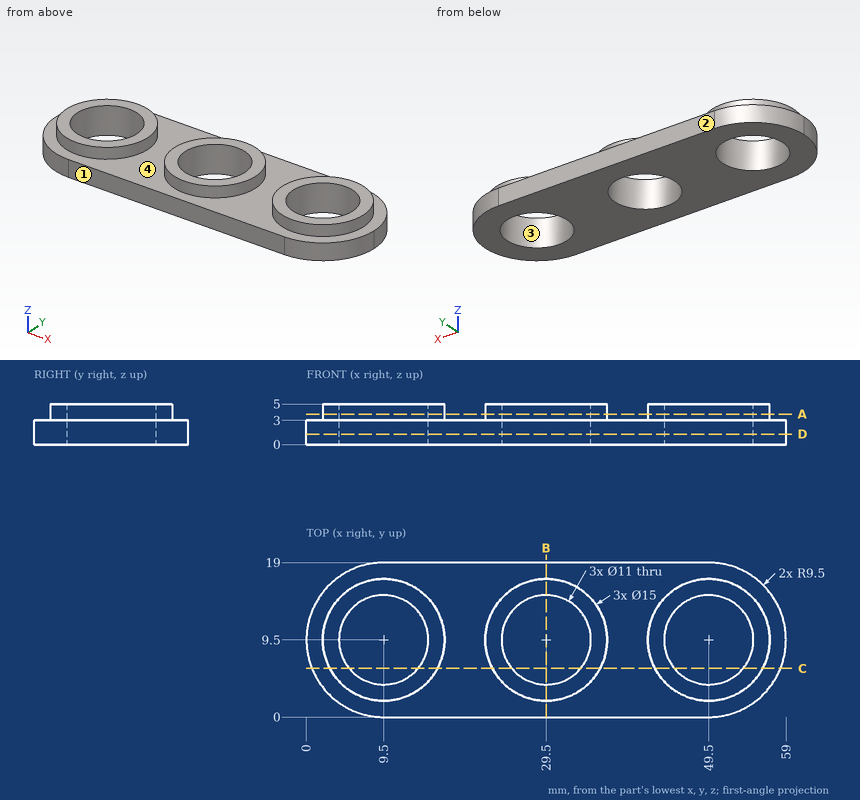
Geometry check sheet. Reference: drawing and pictorial views, mm from the part's lowest x, y, z. Round coordinates to 2 decimals unless told otherwise and drop trailing zeros. Write each loop counter-clockwise with the first axis right and the second up, starting at its lowest first coordinate (ties: lowest second). Pieces come first, ordered by that corner, then holes.
Item 1: Section check D-D (z = 1.3). Record the boundary of the cut face in (x, y), plus the area to 3 significant figures.
Determined:
outline: (9.5, 0) - (49.5, 0) arc R9.5 ccw to (49.5, 19) - (9.5, 19) arc R9.5 ccw to start; hole circle Ø11 at (9.5, 9.5); hole circle Ø11 at (29.5, 9.5); hole circle Ø11 at (49.5, 9.5)
area: 758 mm2
Item 2: Mould release check, pull along Y, two halves, no side actions. Record for the marked faces 1, 2, 3 and 4: +Y half, -Y half, draft (parallel to the pull), parting line (faces both ways), or undercut.
Determined:
face 1: -Y half
face 2: +Y half
face 3: undercut
face 4: draft
Item 3: Section check B-B (x = 29.5). Record the boundary of the cut face in (y, z).
Determined:
outline: (0, 0) - (4, 0) - (4, 5) - (2, 5) - (2, 3) - (0, 3) - close; (15, 0) - (19, 0) - (19, 3) - (17, 3) - (17, 5) - (15, 5) - close
Item 4: Section check C-C (y = 6). Record the boundary of the cut face in (x, z), plus the area to 3 significant figures.
Determined:
outline: (0.67, 0) - (5.26, 0) - (5.26, 5) - (2.87, 5) - (2.87, 3) - (0.67, 3) - close; (13.74, 0) - (25.26, 0) - (25.26, 5) - (22.87, 5) - (22.87, 3) - (16.13, 3) - (16.13, 5) - (13.74, 5) - close; (33.74, 0) - (45.26, 0) - (45.26, 5) - (42.87, 5) - (42.87, 3) - (36.13, 3) - (36.13, 5) - (33.74, 5) - close; (53.74, 0) - (58.33, 0) - (58.33, 3) - (56.13, 3) - (56.13, 5) - (53.74, 5) - close
area: 125 mm2
Item 5: Material ranges on line 1 along Y through (x, z) = (9.5, 2.8); line 2 along X through (y, z) = (5.5, 4.05); line 3 along X through (y, z) = (6.25, 3.65), recorded low to high.
Determined:
line 1: y = 0 to 4, 15 to 19
line 2: x = 3.16 to 5.73, 13.27 to 15.84, 23.16 to 25.73, 33.27 to 35.84, 43.16 to 45.73, 53.27 to 55.84
line 3: x = 2.74 to 5.06, 13.94 to 16.26, 22.74 to 25.06, 33.94 to 36.26, 42.74 to 45.06, 53.94 to 56.26
Item 6: Section check A-A (z = 3.75). Record the boundary of the cut face in (x, y).
Determined:
outline: circle Ø15 at (9.5, 9.5); circle Ø15 at (29.5, 9.5); circle Ø15 at (49.5, 9.5); hole circle Ø11 at (9.5, 9.5); hole circle Ø11 at (29.5, 9.5); hole circle Ø11 at (49.5, 9.5)
